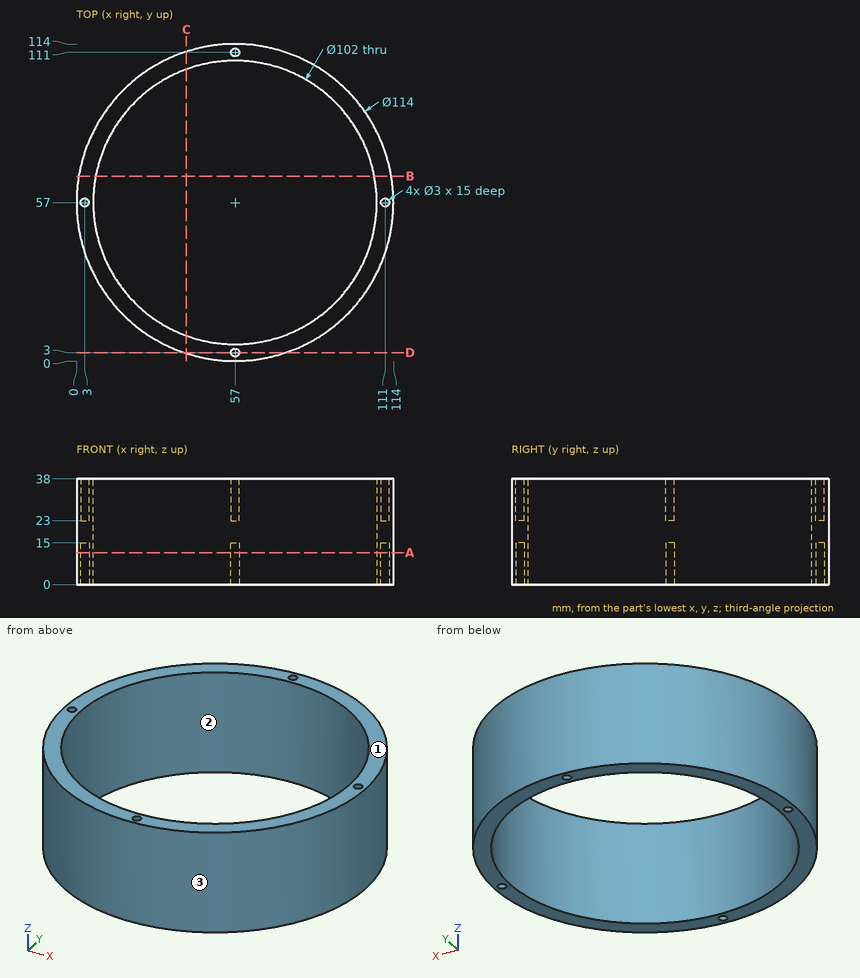
Part print with two shaded views. Sizes in mm from the minimum x, y, z corner. Round coordinates to 2 decimals unless told otherwise and drop trailing zeros. Order: outer loops, then holes, each group sorted by start corner. A loop starts at its lowest first (then second) coordinate and runs counter-clockwise, first axis right, second up. Notation, with made-up numbers: (66, 55) - (78, 55) arc R18 ccw to (78, 76) - close; hole circle Ø7 at (33.5, 41). An arc over 180 degrees is marked (long way). Answer in a Markdown table with one row per item. Add a question column.
(1) Mould opens along Y. For the marked faces 1, 2 and 3 say: +Y half, -Y half, draft (parallel to the pull), parting line (faces both ways), or undercut.
(2) Band-saw the part on D-D on y = 3. List the corners of the cut face in (x, z), and give its area (3 significant figures).
(3) Band-saw the part on A-A on z = 11.5. List the corners of the cut face in (x, y), and give its area (3 significant figures).
(4) Probe L1, parallel to Y at x = 57, z = 10; L2, parallel to X at y = 58, z = 19; L3, parallel to X at y = 27.5, z = 6.5. List the from-to ranges inside material, lowest first. Write a range as [from, to].
(5) Drop flat-ended pins along their axis: pin 1 Ø2.5 at (x, y) = (57, 111) entering from -Z; pin 2 Ø3 at (x, z) = (16, 4) entering from +Y; pin 3 Ø1.5 at (x, y) = (57.5, 2.5) entering from +Z. Give the stop position or say it passes through.
(6) Band-saw the part on B-B on y = 66.5. List the corners of the cut face in (x, z).
(7) Band-saw the part on C-C on x = 39.5. List the corners of the cut face in (y, z), and give its area (3 significant figures).
Data:
| question | item | result |
|---|---|---|
| 1 | face 1 | draft |
| 1 | face 2 | undercut |
| 1 | face 3 | parting line |
| 2 | outline | (38.75, 0) - (55.5, 0) - (55.5, 15) - (58.5, 15) - (58.5, 0) - (75.25, 0) - (75.25, 38) - (58.5, 38) - (58.5, 23) - (55.5, 23) - (55.5, 38) - (38.75, 38) - close |
| 2 | area | 1,300 mm^2 |
| 3 | outline | circle Ø114 at (57, 57); hole circle Ø3 at (3, 57); hole circle Ø102 at (57, 57); hole circle Ø3 at (57, 3); hole circle Ø3 at (57, 111); hole circle Ø3 at (111, 57) |
| 3 | area | 2,010 mm^2 |
| 4 | L1 | y = [0, 1.5], [4.5, 6], [108, 109.5], [112.5, 114] |
| 4 | L2 | x = [0.01, 6.01], [107.99, 113.99] |
| 4 | L3 | x = [8.23, 15.4], [98.6, 105.77] |
| 5 | pin 1 | stops at z = 15 |
| 5 | pin 2 | stops at y = 98.09 |
| 5 | pin 3 | stops at z = 23 |
| 6 | outline | (0.8, 0) - (6.89, 0) - (6.89, 38) - (0.8, 38) - close; (107.11, 0) - (113.2, 0) - (113.2, 38) - (107.11, 38) - close |
| 7 | outline | (2.75, 0) - (9.1, 0) - (9.1, 38) - (2.75, 38) - close; (104.9, 0) - (111.25, 0) - (111.25, 38) - (104.9, 38) - close |
| 7 | area | 482 mm^2 |
